Design review of the part shown in the three views and the two pictorial views. Dimensions are in mm from the part's minimum x, y and z. A direction names the side the tool comes from. Round coordinates to 2 decimals unless told otherwise and drop trailing zeros. Loops run counter-clockwise (first coordinate to the right, second up) from the corner with the lowest first, then second, coordinate; pieces in that order, holes last. Notation, with made-up numbers: (31, 50) -> (54, 50) arc R30 ccw to (54, 76) -> close; hole circle Ø7 at (12, -8). An arc over 180 degrees is marked (long way). Use a Markdown table: item, result. Add a question column.
1) For the marked faces 4, 5 and 6, list the 3-axis set-ups (+Z, -Z, +X, -X, +Y, -Y) from which the entire face can be reached by the end or side of a thin tool; tool diameter is ignored.
2) Mouldability with a two-part tool opening along Z and no side actions: class the marked faces 1, 2 and 3 as released by +Z, released by -Z, zero draft, split by the parting line, or undercut.
3) Consider section A-A on x = 20. Give the boundary of the cut face in (y, z), plus the area to 3 significant figures.
4) Consider section C-C on y = 116. Give the boundary of the cut face in (x, z).
5) Insertion check: pin 1 (9 mm diameter, centred on x = 15.5, z = 21, fed in from +Y); pin 2 (1.5 mm diameter, centred on y = 70, z = 39, fed in from -X); pin 3 (2 mm diameter, centred on x = 32, z = 36.5, fed in from -Y). Each pin has a flat end and moves straight along its axis. Give the tip position at first contact, or say it passes through.
6) Wall thickness on probe 1 along Z at (x, y) = (27, 97.5); probe 2 along Y at (x, z) = (20, 41.25); probe 3 along Y at (x, z) = (20, 38.25): over which ranges is each line inside the solid? List them lowest first.
7) Consider section B-B on y = 103. Give the boundary of the cut face in (x, z).
8) Consider section D-D on z = 25. Give the boundary of the cut face in (x, y).
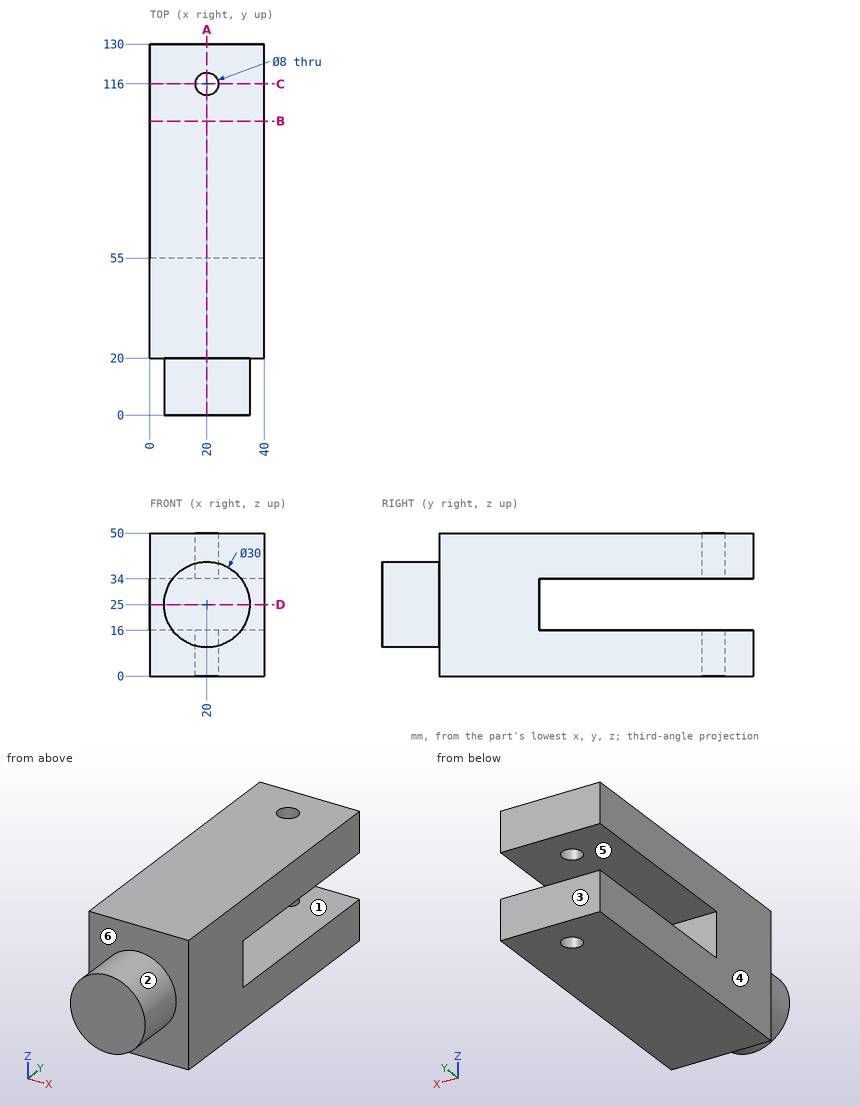
Result set:
| question | item | result |
|---|---|---|
| 1 | face 4 | +Z, -Z, -X, +Y, -Y |
| 1 | face 5 | +X, -X, +Y |
| 1 | face 6 | -Y |
| 2 | face 1 | undercut |
| 2 | face 2 | split by the parting line |
| 2 | face 3 | zero draft |
| 3 | outline | (0, 10) -> (20, 10) -> (20, 0) -> (112, 0) -> (112, 16) -> (55, 16) -> (55, 34) -> (112, 34) -> (112, 50) -> (20, 50) -> (20, 40) -> (0, 40) -> close; (120, 0) -> (130, 0) -> (130, 16) -> (120, 16) -> close; (120, 34) -> (130, 34) -> (130, 50) -> (120, 50) -> close |
| 3 | area | 4,490 mm2 |
| 4 | outline | (0, 0) -> (16, 0) -> (16, 16) -> (0, 16) -> close; (0, 34) -> (16, 34) -> (16, 50) -> (0, 50) -> close; (24, 0) -> (40, 0) -> (40, 16) -> (24, 16) -> close; (24, 34) -> (40, 34) -> (40, 50) -> (24, 50) -> close |
| 5 | pin 1 | y = 55 |
| 5 | pin 2 | x = 0 |
| 5 | pin 3 | y = 20 |
| 6 | probe 1 | 0 to 16, 34 to 50 |
| 6 | probe 2 | 20 to 112, 120 to 130 |
| 6 | probe 3 | 0 to 112, 120 to 130 |
| 7 | outline | (0, 0) -> (40, 0) -> (40, 16) -> (0, 16) -> close; (0, 34) -> (40, 34) -> (40, 50) -> (0, 50) -> close |
| 8 | outline | (0, 20) -> (5, 20) -> (5, 0) -> (35, 0) -> (35, 20) -> (40, 20) -> (40, 55) -> (0, 55) -> close |
